Verification items for the finished model (mm, model axes). Face numbers are marked on the shaded views. Give positions to 0.01 mm unless a question says otherwise; leave off trailing zeros. Loops run counter-clockwise (first coordinate to the right, second up) from the corner with the lowest first, then second, coordinate; pieces in that order, holes last. Notation, with made-up numbers: (-27, 84) - (-22, 84) arc R28 ccw to (-22, 108) - close; hole circle Ø2 at (47, 87.5). An arc over 180 degrees is marked (long way). Answer in a Markdown table with one row per item.
```python
from build123d import *

# Parameters (mm, degrees)
SKETCH_1_R          = 20
EXTRUDE_2_DEPTH     = 10
EXTRUDE_START       = 25
SKETCH_2_R          = 20
SKETCH_2_R_2        = 7
EXTRUDE_3_DEPTH     = 25
SKETCH_3_R          = 3
CUT_EXTRUDE_2_DEPTH = 10
SKETCH_4_R          = 3
CUT_EXTRUDE_3_DEPTH = 20


with BuildPart() as part:
    # 草图1 → 凸台-拉伸2 (new body)
    with BuildSketch(Plane(origin=(0, 0, 0), x_dir=(0, 0, -1), z_dir=(1, 0, 0))):
        Circle(SKETCH_1_R)
    extrude(amount=EXTRUDE_2_DEPTH)

    # 草图2 → 凸台-拉伸3 (add)
    with BuildSketch(Plane.ZY.offset(EXTRUDE_START)):
        Circle(SKETCH_2_R)
        Circle(SKETCH_2_R_2, mode=Mode.SUBTRACT)
    extrude(amount=-EXTRUDE_3_DEPTH)

    # 草图3 → 切除-拉伸2 (cut)
    with BuildSketch(Plane(origin=(10, 0, 0), x_dir=(0, 0, -1), z_dir=(1, 0, 0))):
        Circle(SKETCH_3_R)
    extrude(amount=-CUT_EXTRUDE_2_DEPTH, mode=Mode.SUBTRACT)

    # 草图4 → 切除-拉伸3 (cut, symmetric)
    with BuildSketch(Plane.XY):
        with Locations((-15, 0)):
            Circle(SKETCH_4_R)
    extrude(amount=CUT_EXTRUDE_3_DEPTH, both=True, mode=Mode.SUBTRACT)


solid = part.part
```
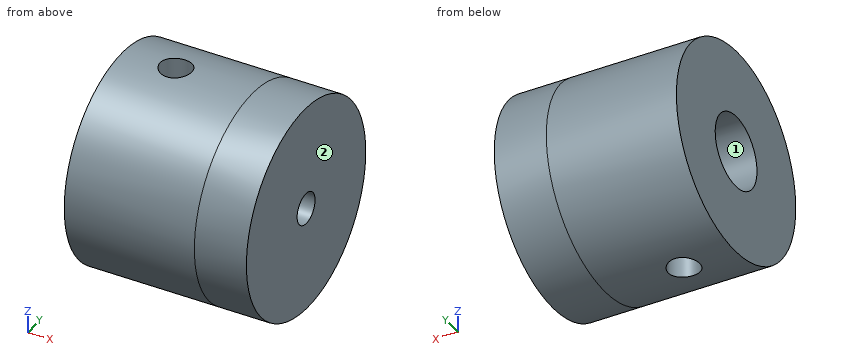
Q1. Thickness scan on line 1 (Y direction, x = -8.5, z = 0); line 2 (Y direction, x = 6, z = 0). Record the ranges inside material, lowest first.
Completed:
| item | result |
|---|---|
| line 1 | -20 to -7, 7 to 20 |
| line 2 | -20 to -3, 3 to 20 |
Q2. Draft check along Z on the marked faces 1 and 2. Enter one of: +Z half, -Z half, draft (parallel to the pull), parting line (faces both ways), or undercut.
Completed:
| item | result |
|---|---|
| face 1 | undercut |
| face 2 | draft |
Q3. Sectioned sample at B-B (y = 0). Record the cut outline in (x, z), and give its area (3 significant figures).
Completed:
| item | result |
|---|---|
| outline | (-25, -20) - (-18, -20) - (-18, -7) - (-25, -7) - close; (-25, 7) - (-18, 7) - (-18, 20) - (-25, 20) - close; (-12, -20) - (10, -20) - (10, -3) - (0, -3) - (0, -7) - (-12, -7) - close; (-12, 7) - (0, 7) - (0, 3) - (10, 3) - (10, 20) - (-12, 20) - close |
| area | 834 mm^2 |
Q4. Sectioned sample at C-C (x = -17). Record the cut outline in (y, z).
Completed:
| item | result |
|---|---|
| outline | (-2.24, -19.87) - (-2.24, -6.63) arc R7 cw to (-2.24, 6.63) - (-2.24, 19.87) arc R20 ccw to start; (2.24, -19.87) arc R20 ccw to (2.24, 19.87) - (2.24, 6.63) arc R7 cw to (2.24, -6.63) - close |
Q5. Sectioned sample at D-D (z = -16). Record the cut outline in (x, y).
Completed:
| item | result |
|---|---|
| outline | (-25, -12) - (10, -12) - (10, 12) - (-25, 12) - close; hole circle Ø6 at (-15, 0) |
Q6. Go/stop test with flat-tipped pins: P1, Ø5, axis at x = -10, z = -1, coming from the +Y side; P2, Ø18, axis at y = 0, z = 0, coming from the +X side; P3, Ø1, axis at y = 0, z = -2, coming from the -X side; P4, Ø4, axis at x = -9.5, y = 3, coming from the -Z side (3 decimals). Record where each tip stops, or that it passes through.
Completed:
| item | result |
|---|---|
| P1 | y = 20 |
| P2 | x = 10 |
| P3 | through |
| P4 | z = -19.975 |
Q7. Sectioned sample at A-A (z = 0). Record the cut outline in (x, y).
Completed:
| item | result |
|---|---|
| outline | (-25, -20) - (10, -20) - (10, -3) - (0, -3) - (0, -7) - (-25, -7) - close; (-25, 7) - (0, 7) - (0, 3) - (10, 3) - (10, 20) - (-25, 20) - close |
